```python
from build123d import *

# Parameters (mm, degrees)
SKETCH1_W                       = 2.499995
SKETCH1_H                       = 8.5000084
SKETCH1_W_2                     = 8.75000028
SKETCH1_H_2                     = 4.499991
TAP_DRILL_FOR_M4X0_7_TAP1_D     = 3.3
TAP_DRILL_FOR_M4X0_7_TAP1_DEPTH = 6.35
TAP_DRILL_FOR_M4X0_7_TAP1_TIP   = 0.991420021


with BuildPart() as part:
    # Sketch1 → Revolve1 (revolve)
    with BuildSketch(Plane.XY, mode=Mode.PRIVATE) as revolve1_sk:
        Polygon((8.75000028, 0), (0, 0), (0, -66.499994), (22.499955, -66.499994), (22.499955, 0), align=None)
        with Locations((1.2499975, 8.7499952)):
            Rectangle(SKETCH1_W, SKETCH1_H)
        with Locations((4.37500014, 2.2499955)):
            Rectangle(SKETCH1_W_2, SKETCH1_H_2)
    revolve(revolve1_sk.sketch.rotate(Axis((0, 8.775492653, 0), (0, -1, 0)), 90), axis=Axis((0, 8.775492653, 0), (0, -1, 0)))

    # Tap Drill for M4x0.7 Tap1
    with Locations(Plane(origin=(0, 0, 0), x_dir=(1, 0, 0), z_dir=(0, 1, 0))):
        with Locations((-14.499971, 0), (14.499971, 0)):
            Hole(TAP_DRILL_FOR_M4X0_7_TAP1_D / 2, depth=TAP_DRILL_FOR_M4X0_7_TAP1_DEPTH)
            with Locations((0, 0, -(TAP_DRILL_FOR_M4X0_7_TAP1_DEPTH + TAP_DRILL_FOR_M4X0_7_TAP1_TIP / 2))):  # 118° drill point
                Cone(0, TAP_DRILL_FOR_M4X0_7_TAP1_D / 2, TAP_DRILL_FOR_M4X0_7_TAP1_TIP, mode=Mode.SUBTRACT)


solid = part.part
```
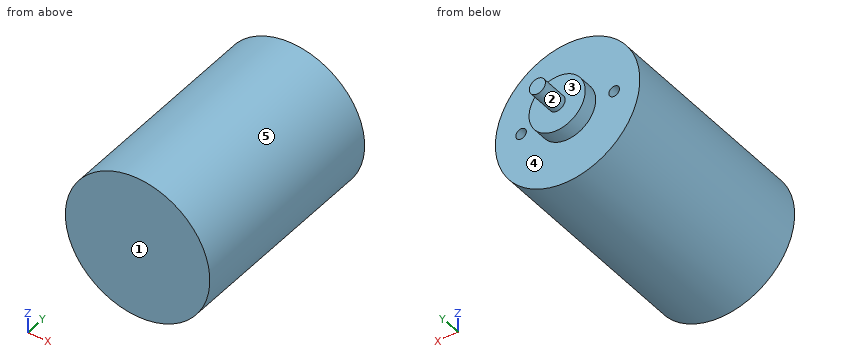
Geometry check sheet. Reference: the model listing, model coordinates, mm. Face numbers are marked on the shaded views. A direction names the side the tool comes from. Round coordinates to 2 decimals unless told otherwise and drop trailing zeros. Order: outer loops, then holes, each group sorted by start corner. A loop starts at its lowest first (then second) coordinate and runs counter-clockwise, first axis right, second up. Notation, with made-up numbers: (-3.75, -14.75) -> (31.25, -14.75) arc R17 ccw to (31.25, 3.25) -> close; hole circle Ø6 at (55, -36.75). An arc over 180 degrees is marked (long way). Return JSON: item names as keys, results as strings. Group by question number.
Q1. Material ranges on probe 1 along Y at (x, z) = (7, -16.5); probe 2 along Z at (x, y) = (-0.5, -63); probe 3 along Z at (x, y) = (-2.5, 1.5), recorded low to high. Write a range as from..to.
Q2. Tool access check on the marked faces 4 and 5. Record the directions out of +Z, -Z, +X, -X, +Y, -Y that give a thin tool (end or side, any length) a straight path to the whole face; none if there is none.
Q3. Section check B-B, the plane z = 6.5. Record the boundary of the cut face in (x, y).
Q4. Section check C-C, the plane y = -51. Record the boundary of the cut face in (x, z), plus the area to 3 significant figures.
Q5. Gauge pin test, flat ends, axial feed: pin 1 (1 mm diameter, centred on y = -1, z = 8, fed in from -X); pin 2 (13.5 mm diameter, centred on x = 9.5, z = 7.5, fed in from +Y); pin 3 (4.5 mm diameter, centred on x = 14.5, z = 0, fed in from +Y); pin 4 (6 mm diameter, centred on y = 4.5, z = 13.5, fed in from +X). Record the tip position at first contact, or that the pin passes through.
Q6. Section check D-D, the plane z = -10.5. Record the boundary of the cut face in (x, y).
Q7. Section check A-A, the plane x = 0. Record the boundary of the cut face in (y, z).
Q8. Release check for a two-part mould opening along Y. For the marked faces 1, 2 and 3 record: released by +Y, released by -Y, zero draft, split by the parting line, or undercut.
Numbers:
{
 "1": {"probe 1": "-66.5..0", "probe 2": "-22.49..22.49", "probe 3": "-8.39..8.39"},
 "2": {"face 4": "+Y", "face 5": "+Y, -Y"},
 "3": {"outline": "(-21.54, -66.5) -> (21.54, -66.5) -> (21.54, 0) -> (5.86, 0) -> (5.86, 4.5) -> (-5.86, 4.5) -> (-5.86, 0) -> (-21.54, 0) -> close"},
 "4": {"outline": "circle Ø45 at (0, 0)", "area": "1,590 mm^2"},
 "5": {"pin 1": "x = -21.21", "pin 2": "y = 4.5", "pin 3": "y = 0", "pin 4": "through"},
 "6": {"outline": "(-19.9, -66.5) -> (19.9, -66.5) -> (19.9, 0) -> (-19.9, 0) -> close"},
 "7": {"outline": "(-66.5, -22.5) -> (0, -22.5) -> (0, -8.75) -> (4.5, -8.75) -> (4.5, -2.5) -> (13, -2.5) -> (13, 2.5) -> (4.5, 2.5) -> (4.5, 8.75) -> (0, 8.75) -> (0, 22.5) -> (-66.5, 22.5) -> close"},
 "8": {"face 1": "released by -Y", "face 2": "zero draft", "face 3": "released by +Y"}
}
